Model file for the job. Use its own axes, mm. Face numbers are marked on the shaded views. A direction names the side the tool comes from. Round coordinates to 2 decimals unless told otherwise and drop trailing zeros. Order: outer loops, then holes, each group sorted by start corner. A loop starts at its lowest first (then second) coordinate and runs counter-clockwise, first axis right, second up. Notation, with made-up numbers: (84, -20) -> (115, -20) arc R23 ccw to (115, -4) -> close; hole circle Ø1 at (69, 21). An arc over 180 degrees is marked (long way). Answer as CSV lines item,"result".
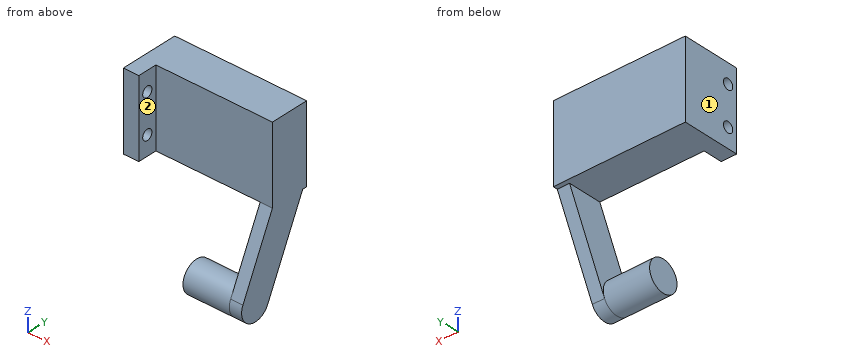
```python
from build123d import *

# Parameters (mm, degrees)
SKETCH1_W           = 20
SKETCH1_H           = 15
SKETCH1_R           = 1.35
BOSS_EXTRUDE1_DEPTH = 4
SKETCH2_W           = 20
SKETCH2_H           = 10
BOSS_EXTRUDE2_DEPTH = 27
BOSS_EXTRUDE3_DEPTH = 3.175
BOSS_EXTRUDE4_START = 12
SKETCH4_R           = 4
BOSS_EXTRUDE4_DEPTH = 12


with BuildPart() as part:
    # Sketch1 → Boss-Extrude1 (new body)
    with BuildSketch(Plane(origin=(0, 0, 0), x_dir=(0, 0, -1), z_dir=(1, 0, 0))):
        Rectangle(SKETCH1_W, SKETCH1_H)
        with Locations((-5, -5)):
            Circle(SKETCH1_R, mode=Mode.SUBTRACT)
        with Locations((5, -5)):
            Circle(SKETCH1_R, mode=Mode.SUBTRACT)
    extrude(amount=BOSS_EXTRUDE1_DEPTH)

    # Sketch2 → Boss-Extrude2 (add)
    with BuildSketch(Plane(origin=(4, 0, 0), x_dir=(0, 0, -1), z_dir=(1, 0, 0))):
        with Locations((0, 2.5)):
            Rectangle(SKETCH2_W, SKETCH2_H)
    extrude(amount=BOSS_EXTRUDE2_DEPTH)

    # Sketch3 → Boss-Extrude3 (add)
    with BuildSketch(Plane(origin=(31, 0, 0), x_dir=(0, 0, -1), z_dir=(1, 0, 0))):
        with BuildLine():
            Line((10, 7.5), (-10, 7.5))
            Line((-10, 7.5), (-10, -2.5))
            Line((-10, -2.5), (10, -2.5))
            Line((10, -2.5), (28.295353016, -11.118587937))
            ThreePointArc((28.295353016, -11.118587937), (33.618587937, -9.204646984), (31.704646984, -3.881412063))
            Line((31.704646984, -3.881412063), (10, 6.343228507))
            Line((10, 6.343228507), (10, 7.5))
        make_face()
    extrude(amount=BOSS_EXTRUDE3_DEPTH)

    # Sketch4 → Boss-Extrude4 (add)
    with BuildSketch(Plane.ZY.offset(-31).offset(BOSS_EXTRUDE4_START)):
        with Locations((-30, -7.5)):
            Circle(SKETCH4_R)
    extrude(amount=-BOSS_EXTRUDE4_DEPTH)


solid = part.part
```
Q1. Saw through at A-A (z = -5). Write the cut outline in (x, y) (3 decimals).
Checks:
outline,"(0, -7.5) -> (4, -7.5) -> (4, -6.35) -> (0, -6.35) -> close; (0, -3.65) -> (4, -3.65) -> (4, -2.5) -> (34.175, -2.5) -> (34.175, 7.5) -> (0, 7.5) -> close"
Q2. Tool access for the marked faces 1 and 2: list every direction of +Z, -Z, +X, -X, +Y, -Y with a clear straight run to the whole face (end or side of a thin tool).
Checks:
face 1,"+Z, -Z, -X, +Y, -Y"
face 2,"+Z, -Z, +X, -Y"
Q3. Wall check: L1, parallel to X at y = -2, z = -23 (3 decimals); L2, parallel to Z at x = 13, y = -1.5; L3, parallel to X at y = -6, z = -1.5. Give the ranges that are in metal, low to high. Write a range as [from, to].
Checks:
L1,"[31, 34.175]"
L2,"[-10, 10]"
L3,"[0, 4]"
Q4. Saw through at B-B (x = 3.5). Write the cut outline in (y, z).
Checks:
outline,"(-7.5, -10) -> (7.5, -10) -> (7.5, 10) -> (-7.5, 10) -> close; hole circle Ø2.7 at (-5, -5); hole circle Ø2.7 at (-5, 5)"
Q5. Saw through at C-C (y = -5). State how many separate pieces and enclosed holes the cut face has, plus the area to 3 significant figures.
Checks:
separate pieces,"4"
enclosed holes,"0"
area,"190 mm²"
Q6. Flat gauge pins, fed straight in: pin 1 (2 mm diameter, centred on x = 2.5, z = 3.5, fed in from -Y); pin 2 (8 mm diameter, centred on x = 22, y = 2, fed in from -Z); pin 3 (9 mm diameter, centred on y = -6.5, z = -32, fed in from -X); pin 4 (5 mm diameter, centred on y = 0.5, z = -1.5, fed in from -X). Where does each tip first touch, or does it go through?
Checks:
pin 1,"y = -7.5"
pin 2,"z = -10"
pin 3,"x = 19"
pin 4,"x = 0"
Q7. Saw through at D-D (y = -0.5). Write the cut outline in (x, z) (3 decimals), plus the area to 3 significant figures.
Checks:
outline,"(0, -10) -> (31, -10) -> (31, -24.527) -> (34.175, -24.527) -> (34.175, 10) -> (0, 10) -> close"
area,"730 mm²"
